```python
from build123d import *

# Parameters (mm, degrees)
SKETCH1_R           = 3.175
BOSS_EXTRUDE1_DEPTH = 5.461
SKETCH2_W           = 4.7625
SKETCH2_H           = 33.783
CUT_EXTRUDE1_DEPTH  = 6.461


with BuildPart() as part:
    # Sketch1 → Boss-Extrude1 (new body)
    with BuildSketch(Plane(origin=(0, 0, 0), x_dir=(1, 0, 0), z_dir=(0, 1, 0))):
        with BuildLine():
            Line((-82.674132744, 104.451069294), (-69.310188895, 104.451069294))
            ThreePointArc((-69.310188895, 104.451069294), (-55.336180049, 99.157726681), (-42.113057451, 106.117714323))
            Line((-42.113057451, 106.117714323), (0, 94.833554589))
            Line((0, 94.833554589), (0, 58.293))
            Line((0, 58.293), (8, 58.293))
            Line((8, 58.293), (8, -58.293))
            Line((8, -58.293), (0, -58.293))
            Line((0, -58.293), (0, -94.833554589))
            Line((0, -94.833554589), (-42.113057451, -106.117714323))
            ThreePointArc((-42.113057451, -106.117714323), (-55.336180049, -99.157726681), (-69.310188895, -104.451069294))
            Line((-69.310188895, -104.451069294), (-82.674132744, -104.451069294))
            ThreePointArc((-82.674132744, -104.451069294), (-86.841727728, -94.209575285), (-83.629476528, -83.629476528))
            Line((-83.629476528, -83.629476528), (0, 0))
            Line((0, 0), (-83.629476528, 83.629476528))
            ThreePointArc((-83.629476528, 83.629476528), (-86.841727728, 94.209575285), (-82.674132744, 104.451069294))
        make_face()
        with Locations((-70.310188895, 93.451069294)):
            Circle(SKETCH1_R, mode=Mode.SUBTRACT)
        with Locations((-70.310188895, -93.451069294)):
            Circle(SKETCH1_R, mode=Mode.SUBTRACT)
    extrude(amount=BOSS_EXTRUDE1_DEPTH)

    # Sketch2 → Cut-Extrude1 (cut, through all)
    with BuildSketch(Plane(origin=(0, 0, 0), x_dir=(1, 0, 0), z_dir=(0, 1, 0))):
        Polygon((-17.19282542, -99.440358276), (-4.829629131, -96.127649814), (-6.062254834, -91.527428067), (-18.425451123, -94.840136528), align=None)
        Polygon((-37.283428319, -104.823619098), (-24.920232031, -101.510910637), (-26.152857733, -96.910688889), (-38.516054022, -100.22339735), align=None)
        with Locations((5.61875, -33.4015)):
            Rectangle(SKETCH2_W, SKETCH2_H)
        Polygon((-38.516054022, 100.22339735), (-26.152857733, 96.910688889), (-24.920232031, 101.510910637), (-37.283428319, 104.823619098), align=None)
        Polygon((-18.425451123, 94.840136528), (-6.062254834, 91.527428067), (-4.829629131, 96.127649814), (-17.19282542, 99.440358276), align=None)
        with Locations((5.61875, 33.4015)):
            Rectangle(SKETCH2_W, SKETCH2_H)
    extrude(amount=CUT_EXTRUDE1_DEPTH, mode=Mode.SUBTRACT)


solid = part.part
```
Here's how the part is built. I have some questions about the finished solid (model axes, mm). A direction names the side the tool comes from. Give positions to 0.01 mm unless a question says otherwise; leave off trailing zeros. Order: outer loops, then holes, each group sorted by start corner. A loop starts at its lowest first (then second) coordinate and runs counter-clockwise, first axis right, second up. Notation, with made-up numbers: (60.25, 19) -> (106.25, 19) arc R19 ccw to (106.25, 51) -> close; hole circle Ø2 at (-34.5, 58). An arc over 180 degrees is marked (long way). Use CSV: the item, a comma, the result in double quotes. Start each with the question number.
Item 1: Thinking about a two-plate mould opening in Z: for faces 6 (the flat face through (8, 3, 54)), 7 (the cylindrical face through (-86.834, 2.692, 94.367)), 8 (the flat face through (-76, 3, -104.451)), which applies, pulls with the +Z half, pulls with the -Z half, needs draft (parallel to the pull), parting line crosses it, or undercut?
Item 2: I'm going to push flat-ended pins straight in: P1, Ø2.5, axis at y = 3, z = -31, coming from the +X side; P2, Ø1.6, axis at x = -73.5, y = 2.5, coming from the -Z side; P3, Ø1, axis at y = 1, z = -66, coming from the -X side. Where does each tip first touch, or does it pass through?
Item 3: On a 3-axis mill with a long thin cutter (end or side, diameter ignored), from which of +Z, -Z, +X, -X, +Y, -Y can I reach the whole of each face in a straight line? I mean faces 1 (the flat face through (6, 3, -16.51)), 2 (the flat face through (-25.53, 2.69, 99.24)), 3 (the flat face through (-5.455, 2.692, -93.795)), 4 (the flat face through (0, 3, -77)), 5 (the flat face through (-42, 3, 42)). Say none if no direction works.
Item 4: If I drill on probe 1 along Z at (x, y) = (-71.5, 1.1); probe 2 along Z at (x, y) = (-74, 2.95); probe 3 along Z at (x, y) = (-14.5, 2.2), over which ranges is the centre line in solid material (lowest first)? Write a range as [from, to].
Item 5: Suppose I cut it at A-A (x = -58). List the corners of the cut face in (y, z) for me, and give its area (3 significant figures).
Item 6: Suppose I cut it at D-D (z = 47.5). List the corners of the cut face in (x, y) for me.
Item 7: Suppose I cut it at C-C (y = 2.95). Give the number of separate pieces and of enclosed holes in the cut face, and give its area (3 significant figures).
Item 8: Suppose I cut it at B-B (z = 2). List the corners of the cut face in (x, y) for me.
Answer block:
1,face 6,"needs draft"
1,face 7,"undercut"
1,face 8,"pulls with the -Z half"
2,P1,"stops at x = 3.24"
2,P2,"stops at z = -104.45"
2,P3,"stops at x = -66.5"
3,face 1,"+X, +Y, -Y"
3,face 2,"+Z, +Y, -Y"
3,face 3,"-Z, +Y, -Y"
3,face 4,"-Z, +X, +Y, -Y"
3,face 5,"-X, +Y, -Y"
4,probe 1,"z = [-104.45, -96.39], [-90.51, -71.5], [71.5, 90.51], [96.39, 104.45]"
4,probe 2,"z = [-104.45, -74], [74, 104.45]"
4,probe 3,"z = [-93.79, -14.5], [14.5, 93.79]"
5,outline,"(0, -99.19) -> (5.46, -99.19) -> (5.46, -58) -> (0, -58) -> close; (0, 58) -> (5.46, 58) -> (5.46, 99.19) -> (0, 99.19) -> close"
5,area,"450 mm^2"
6,outline,"(-47.5, 0) -> (3.24, 0) -> (3.24, 5.46) -> (-47.5, 5.46) -> close"
7,separate pieces,"1"
7,enclosed holes,"2"
7,area,"10,300 mm^2"
8,outline,"(-2, 0) -> (8, 0) -> (8, 5.46) -> (-2, 5.46) -> close"
